```python
from build123d import *

# Parameters (mm, degrees)
F0_R      = 55
F1_DEPTH  = 25
F2_SIZE2  = 20
F2_SIZE   = 22.5
F3_R      = 27.5
F4_DEPTH  = 20
F6_START  = -5
F5_R      = 32.5
F5_R_2    = 27.5
F6_DEPTH  = 10
F7_R      = 65
F8_DEPTH  = 3
F9_R      = 2
F10_DEPTH = 25
F11_R     = 45
F12_DEPTH = 15
F12_TAPER = 60
F13_DEPTH = 10
F15_R     = 55
F15_R_2   = 45
F16_DEPTH = 4


# Not quite as in the source:
# - a fillet or chamfer that OpenCascade refuses, or shapes differently, is made with other operations: its cross-section is extruded or revolved along the edge and cut away or added


with BuildPart() as f1:
    # F0 (on Front) → F1 (new body)
    with BuildSketch(Plane.XZ):
        Circle(F0_R)
    extrude(amount=F1_DEPTH)

    # F2
    f2_edges = [f1.edges().sort_by_distance(p)[0] for p in [
        (-55, -25, 0),
    ]]
    f2_side = f1.faces().sort_by_distance((0, -25, 0))[0]
    chamfer(f2_edges, length=F2_SIZE, length2=F2_SIZE2, reference=f2_side)

    # F3 (on face) → F4 (join)
    with BuildSketch(Plane.XZ.offset(25)):
        Circle(F3_R)
    extrude(amount=F4_DEPTH)

    # F5 (on face) → F6 (join)
    with BuildSketch(Plane.XZ.offset(45).offset(F6_START)):
        Circle(F5_R)
        Circle(F5_R_2, mode=Mode.SUBTRACT)
    extrude(amount=-F6_DEPTH)

    # F7 (on face) → F8 (join)
    with BuildSketch(Plane(origin=(0, 0, 0), x_dir=(-1, 0, 0), z_dir=(0, 1, 0))):
        Circle(F7_R)
    extrude(amount=F8_DEPTH)

    # F9 (on face) → F10 (cut)
    with BuildSketch(Plane(origin=(0, 3, 0), x_dir=(-1, 0, 0), z_dir=(0, 1, 0))):
        with Locations((-42.5, 42.5)):
            Circle(F9_R)
        with Locations((42.5, 42.5)):
            Circle(F9_R)
        with Locations((42.5, -42.5)):
            Circle(F9_R)
        with Locations((-42.5, -42.5)):
            Circle(F9_R)
    extrude(amount=-F10_DEPTH, mode=Mode.SUBTRACT)

    # F11 (on face) → F12 (cut)
    with BuildSketch(Plane(origin=(0, 3, 0), x_dir=(-1, 0, 0), z_dir=(0, 1, 0))):
        Circle(F11_R)
    extrude(amount=-F12_DEPTH, taper=F12_TAPER, mode=Mode.SUBTRACT)

    # F13 (add): a face of the model
    f13_faces = [f1.faces().sort_by_distance(p)[0] for p in [
        (0, -12, 0),
    ]]
    extrude(f13_faces, amount=F13_DEPTH)

    # F14: fillet of radius 23 on 1 edges, made by hand

    # F14_s1 → F14_t2 (revolve, cut)
    with BuildSketch(Plane.XY):
        with BuildLine():
            ThreePointArc((-19.0192378865, -12), (-10.7693772202, -4.6530100506), (-0.0455719255, -2))
            Line((-0.0455719255, -2), (-19.0192378865, -2))
            Line((-19.0192378865, -2), (-19.0192378865, -12))
        make_face()
    revolve(axis=Axis((0, -2, 0), (0, 1, 0)), mode=Mode.SUBTRACT)

    # F15 (on face) → F16 (join)
    with BuildSketch(Plane(origin=(0, 3, 0), x_dir=(-1, 0, 0), z_dir=(0, 1, 0))):
        Circle(F15_R)
        Circle(F15_R_2, mode=Mode.SUBTRACT)
    extrude(amount=F16_DEPTH)

    # F17: fillet of radius 5.1 on 2 edges, made by hand

    # F17_s1 → F17_t2 (revolve, cut)
    with BuildSketch(Plane.XY):
        with BuildLine():
            ThreePointArc((-55, 3), (-53.2137840453, 5.8761790704), (-50.0200401608, 7))
            Line((-50.0200401608, 7), (-55, 7))
            Line((-55, 7), (-55, 3))
        make_face()
    revolve(axis=Axis((0, 7, 0), (0, 1, 0)), mode=Mode.SUBTRACT)

    # F17_s3 → F17_t4 (revolve, cut)
    with BuildSketch(Plane.XY):
        with BuildLine():
            ThreePointArc((-49.9799598392, 7), (-46.7862159547, 5.8761790704), (-45, 3))
            Line((-45, 3), (-45, 7))
            Line((-45, 7), (-49.9799598392, 7))
        make_face()
    revolve(axis=Axis((0, 7, 0), (0, 1, 0)), mode=Mode.SUBTRACT)


solid = f1.part
```
For this review, take the finished solid that the model builds, in its own axes (mm). A direction names the side the tool comes from. Round coordinates to 2 decimals unless told otherwise and drop trailing zeros. Write each loop counter-clockwise with the first axis right and the second up, starting at its lowest first coordinate (ties: lowest second). Pieces come first, ordered by that corner, then holes. Notation, with made-up numbers: (-8.75, -10) - (23.25, -10) arc R20 cw to (23.25, -4) - close; hole circle Ø10 at (48.25, 71.5). An arc over 180 degrees is marked (long way). Put each result on its own line as item: value.
Q1. Insertion check: pin 1 Ø2 at (x, z) = (19.5, 43.5) entering from +Y; pin 2 Ø1.5 at (y, z) = (-4, -8.5) entering from +X; pin 3 Ø5 at (x, z) = (35, -26) entering from +Y. Each pin has a flat end and moves straight along its axis. Give the tip position at first contact, or say it passes through.
Solved:
pin 1: stops at y = 6.83
pin 2: stops at x = 54.45
pin 3: stops at y = 5.21
Q2. Wall thickness on probe 1 along Y at (x, z) = (27.5, -53.5); probe 2 along X at (y, z) = (1, -42); probe 3 along Y at (x, z) = (-20, -22.5): over which ranges is each line inside the solid? List them lowest first.
Solved:
probe 1: y = 0 to 3
probe 2: x = -49.61 to -44.44, -40.56 to 40.56, 44.44 to 49.61
probe 3: y = -40 to -30, -25 to -5.6
Q3. Machinability: for faces 5 (the face through (-5.961, -27.465, -26.846)), 6 (the face through (29, 3, -48)), 7 (the face through (-5.961, -42.465, -26.846)), 8 (the face through (42.934, 1.521, 40.548)), 9 (the face through (0, -45, 0)), which of the approach directions +Z, -Z, +X, -X, +Y, -Y give a long, thin tool a straight path to every point of the face, cutting with its end or side? Answer none if there is none.
Solved:
face 5: none
face 6: +Y
face 7: -Y
face 8: +Y, -Y
face 9: +Z, -Z, +X, -X, -Y
Q4. Mouldability with a two-part tool opening along Z and no side actions: class faces 1 (the face through (-18.734, -11.272, -7.768)), 2 (the face through (31, -35.07, 9.76)), 3 (the face through (-42.066, 1.521, -44.452)), 4 (the face through (29, 0, -48)) as released by +Z, released by -Z, zero draft, split by the parting line, or undercut.
Solved:
face 1: undercut
face 2: split by the parting line
face 3: undercut
face 4: zero draft
Q5. We need section B-B (x = -42.5). Count the separate pieces of the cut face and the enclosed holes in it, and give its area (3 significant figures).
Solved:
separate pieces: 3
enclosed holes: 0
area: 1,210 mm2
Q6. We need section A-A (y = -15). Give the boundary of the cut face in (x, z).
Solved:
outline: circle Ø87.5 at (0, 0)
